```python
from build123d import *

# Parameters (mm, degrees)
EXTRUDE_1_DEPTH     = 2.121152063
SKETCH_2_W          = 18.284159781
SKETCH_2_H          = 2.121152063
EXTRUDE_2_DEPTH     = 1.283615947
SKETCH_3_W          = 7.715840219
SKETCH_3_H          = 2.121152063
EXTRUDE_3_DEPTH     = 1.283615947
EXTRUDE_4_DEPTH     = 4.2
SKETCH_5_W          = 31.999368794
SKETCH_5_H          = 4.790748137
EXTRUDE_5_DEPTH     = 2.1
SKETCH_6_W          = 12.000251863
SKETCH_6_H          = 4.2
CUT_EXTRUDE_1_DEPTH = 2.32
CUT_EXTRUDE_2_DEPTH = 23.550749058
EXTRUDE_6_DEPTH     = 3.1
EXTRUDE_7_DEPTH     = 3.1
CUT_EXTRUDE_3_DEPTH = 1
CUT_EXTRUDE_4_DEPTH = 2.6
CUT_EXTRUDE_5_DEPTH = 2.6
CUT_EXTRUDE_6_DEPTH = 0.7
CUT_EXTRUDE_7_DEPTH = 3.090748137
CUT_EXTRUDE_8_DEPTH = 3.090748137
HOLE_WIZARD_1_D     = 2.4
HOLE_WIZARD_1_DEPTH = 16.79105
HOLE_WIZARD_2_D     = 2.4
HOLE_WIZARD_2_DEPTH = 16.79105
HOLE_WIZARD_3_D     = 2.4
HOLE_WIZARD_3_DEPTH = 16.79105
HOLE_WIZARD_4_D     = 2.4
HOLE_WIZARD_4_DEPTH = 16.79105
FILLET_1_R          = 1
FILLET_2_R          = 1
FILLET_3_R          = 1
FILLET_4_R          = 1
FILLET_5_R          = 3
FILLET_6_R          = 3


with BuildPart() as part:
    # ｽｹｯﾁ1 → ﾎﾞｽ - 押し出し1 (new body)
    with BuildSketch(Plane.XZ.offset(24)):
        with BuildLine():
            Line((-17, 4.6), (-17, -10.907384053))
            Line((-17, -10.907384053), (1.284159781, -10.907384053))
            Line((1.284159781, -10.907384053), (1.284159781, -9.036499448))
            ThreePointArc((1.284159781, -9.036499448), (-3.636777298, -7.097679354), (-0.031629692, -3.227594621))
            ThreePointArc((-0.031629692, -3.227594621), (9.064370854, -1.683948584), (9.284159781, -10.907384053))
            Line((9.284159781, -10.907384053), (17, -10.907384053))
            Line((17, -10.907384053), (17, 4.6))
            Line((17, 4.6), (-17, 4.6))
        make_face()
    extrude(amount=-EXTRUDE_1_DEPTH)

    # ｽｹｯﾁ2 → ﾎﾞｽ - 押し出し2 (add)
    with BuildSketch(Plane(origin=(0, 0, -10.907384053), x_dir=(-1, 0, 0), z_dir=(0, 0, -1))):
        with Locations((7.85792011, -22.939423969)):
            Rectangle(SKETCH_2_W, SKETCH_2_H)
    extrude(amount=EXTRUDE_2_DEPTH)

    # ｽｹｯﾁ3 → ﾎﾞｽ - 押し出し3 (add)
    with BuildSketch(Plane(origin=(0, 0, -10.907384053), x_dir=(-1, 0, 0), z_dir=(0, 0, -1))):
        with Locations((-13.14207989, -22.939423969)):
            Rectangle(SKETCH_3_W, SKETCH_3_H)
    extrude(amount=EXTRUDE_3_DEPTH)

    # ｽｹｯﾁ4 → ﾎﾞｽ - 押し出し4 (add)
    with BuildSketch(Plane(origin=(0, -21.878847937, 0), x_dir=(-1, 0, 0), z_dir=(0, 1, 0))):
        with BuildLine():
            Line((17, 4.6), (17, -12.191))
            Line((17, -12.191), (11.515840219, -12.191))
            Line((11.515840219, -12.191), (11.515840219, -0.190748137))
            Line((11.515840219, -0.190748137), (-9.284159781, -0.190748137))
            Line((-9.284159781, -0.190748137), (-9.284159781, -12.191))
            add(Edge.make_bspline(
                [(-9.284159781, -12.191), (-10.057493115, -12.191), (-10.830826448, -12.191), (-11.604159781, -12.191)],
                knots=[0, 0, 0, 0, 1, 1, 1, 1], degree=3))
            Line((-11.604159781, -12.191), (-17, -12.191))
            Line((-17, -12.191), (-17, 4.6))
            Line((-17, 4.6), (17, 4.6))
        make_face()
    extrude(amount=EXTRUDE_4_DEPTH)

    # ｽｹｯﾁ5 → ﾎﾞｽ - 押し出し5 (add)
    with BuildSketch(Plane(origin=(0, -17.678847937, 0), x_dir=(-1, 0, 0), z_dir=(0, 1, 0))):
        with Locations((-0.000159781, 2.204625932)):
            Rectangle(SKETCH_5_W, SKETCH_5_H)
    extrude(amount=EXTRUDE_5_DEPTH)

    # ｽｹｯﾁ6 → ｶｯﾄ - 押し出し1 (cut)
    with BuildSketch(Plane.ZY.offset(-9.284159781)):
        with Locations((-6.190874069, -19.778847937)):
            Rectangle(SKETCH_6_W, SKETCH_6_H)
    extrude(amount=-CUT_EXTRUDE_1_DEPTH, mode=Mode.SUBTRACT)

    # ｽｹｯﾁ7 → ｶｯﾄ - 押し出し2 (cut, through all)
    with BuildSketch(Plane.XZ.offset(24)):
        with BuildLine():
            Line((1.284159781, -11.081163897), (1.284159781, -9.036499448))
            ThreePointArc((1.284159781, -9.036499448), (0.655198078, -9.368779249), (-0.031629692, -9.553901653))
            ThreePointArc((-0.031629692, -9.553901653), (0.562738255, -10.37226331), (1.284159781, -11.081163897))
        make_face()
    extrude(amount=-CUT_EXTRUDE_2_DEPTH, mode=Mode.SUBTRACT)

    # ｽｹｯﾁ8 → ﾎﾞｽ - 押し出し6 (add)
    with BuildSketch(Plane(origin=(0, -17.678847937, 0), x_dir=(-1, 0, 0), z_dir=(0, 1, 0))):
        with BuildLine():
            Line((15.999524616, -6.990748137), (14.777524616, -6.990748137))
            ThreePointArc((14.777524616, -6.990748137), (12.865840219, -6.390748137), (14.777524616, -5.790748137))
            Line((14.777524616, -5.790748137), (15.999524616, -5.790748137))
            Line((15.999524616, -5.790748137), (15.999524616, -6.990748137))
        make_face()
    extrude(amount=EXTRUDE_6_DEPTH)

    # ｽｹｯﾁ9 → ﾎﾞｽ - 押し出し7 (add)
    with BuildSketch(Plane(origin=(0, -17.678847937, 0), x_dir=(-1, 0, 0), z_dir=(0, 1, 0))):
        with BuildLine():
            Line((-15.999844178, -5.790748137), (-14.745844178, -5.790748137))
            ThreePointArc((-14.745844178, -5.790748137), (-12.834159781, -6.390748137), (-14.745844178, -6.990748137))
            Line((-14.745844178, -6.990748137), (-15.999844178, -6.990748137))
            Line((-15.999844178, -6.990748137), (-15.999844178, -5.790748137))
        make_face()
    extrude(amount=EXTRUDE_7_DEPTH)

    # ｽｹｯﾁ10 → ｶｯﾄ - 押し出し3 (cut)
    with BuildSketch(Plane.XY.offset(4.6)):
        Polygon((-0.599999987, -17.799999602), (-2.834665696, -19.9353347), (-0.599999987, -22.159852817), (-0.599999987, -20.818248187), (2.589334329, -20.818248187), (2.589334329, -18.999999575), (-0.599999987, -18.999999575), align=None)
    extrude(amount=-CUT_EXTRUDE_3_DEPTH, mode=Mode.SUBTRACT)

    # ｽｹｯﾁ11 → ｶｯﾄ - 押し出し4 (cut)
    with BuildSketch(Plane.XY.offset(4.6)):
        Polygon((-14.535820787, -22.230633649), (-12.22641971, -22.230633649), (-11.071719172, -20.230633649), (-12.22641971, -18.230633649), (-14.535820787, -18.230633649), (-15.690521325, -20.230633649), align=None)
    extrude(amount=-CUT_EXTRUDE_4_DEPTH, mode=Mode.SUBTRACT)

    # ｽｹｯﾁ12 → ｶｯﾄ - 押し出し5 (cut)
    with BuildSketch(Plane.XY.offset(4.6)):
        Polygon((12.255035689, -22.231967066), (14.564436765, -22.231967066), (15.719137304, -20.231967066), (14.564436765, -18.231967066), (12.255035689, -18.231967066), (11.10033515, -20.231967066), align=None)
    extrude(amount=-CUT_EXTRUDE_5_DEPTH, mode=Mode.SUBTRACT)

    # ｽｹｯﾁ13 → ｶｯﾄ - 押し出し6 (cut)
    with BuildSketch(Plane(origin=(0, -21.878847937, 0), x_dir=(-1, 0, 0), z_dir=(0, 1, 0))):
        Polygon((7.518980495, -7.752475082), (5.003355584, -7.752475082), (5.003355584, -8.596713483), (8.530699304, -8.596713483), (8.530699304, -3.62698698), (7.518980495, -3.62698698), align=None)
    extrude(amount=-CUT_EXTRUDE_6_DEPTH, mode=Mode.SUBTRACT)

    # ｽｹｯﾁ14 → ｶｯﾄ - 押し出し7 (cut)
    with BuildSketch(Plane(origin=(0, 0, -0.190748137), x_dir=(-1, 0, 0), z_dir=(0, 0, -1))):
        Polygon((-7.185754105, -20.683997984), (-4.876353029, -20.683997984), (-3.72165249, -18.683997984), (-4.876353029, -16.683997984), (-7.185754105, -16.683997984), (-8.340454644, -18.683997984), align=None)
    extrude(amount=-CUT_EXTRUDE_7_DEPTH, mode=Mode.SUBTRACT)

    # ｽｹｯﾁ15 → ｶｯﾄ - 押し出し8 (cut)
    with BuildSketch(Plane(origin=(0, 0, -0.190748137), x_dir=(-1, 0, 0), z_dir=(0, 0, -1))):
        Polygon((4.835886318, -20.763995351), (7.145287395, -20.763995351), (8.299987933, -18.763995351), (7.145287395, -16.763995351), (4.835886318, -16.763995351), (3.68118578, -18.763995351), align=None)
    extrude(amount=-CUT_EXTRUDE_8_DEPTH, mode=Mode.SUBTRACT)

    # 穴1
    with Locations(Plane.XY.offset(4.6)):
        with Locations((-5.97769389, -18.770751676)):
            Hole(HOLE_WIZARD_1_D / 2, depth=HOLE_WIZARD_1_DEPTH)

    # 穴2
    with Locations(Plane.XY.offset(4.6)):
        with Locations((6.022013453, -18.686944197)):
            Hole(HOLE_WIZARD_2_D / 2, depth=HOLE_WIZARD_2_DEPTH)

    # 穴3
    with Locations(Plane(origin=(0, 0, -12.191), x_dir=(-1, 0, 0), z_dir=(0, 0, -1))):
        with Locations((-13.4, -20.25)):
            Hole(HOLE_WIZARD_3_D / 2, depth=HOLE_WIZARD_3_DEPTH)

    # 穴4
    with Locations(Plane(origin=(0, 0, -12.191), x_dir=(-1, 0, 0), z_dir=(0, 0, -1))):
        with Locations((13.4, -20.25)):
            Hole(HOLE_WIZARD_4_D / 2, depth=HOLE_WIZARD_4_DEPTH)

    # ﾌｨﾚｯﾄ1
    fillet_1_edges = [part.edges().sort_by_distance(p)[0] for p in [
        (9.284159781, -22.939423968, -10.907384053),
    ]]
    fillet(fillet_1_edges, radius=FILLET_1_R)

    # ﾌｨﾚｯﾄ2
    fillet_2_edges = [part.edges().sort_by_distance(p)[0] for p in [
        (1.284159781, -22.939423968, -11.081163897),
    ]]
    fillet(fillet_2_edges, radius=FILLET_2_R)

    # ﾌｨﾚｯﾄ3
    fillet_3_edges = [part.edges().sort_by_distance(p)[0] for p in [
        (-17, -17.678847937, -3.7955),
    ]]
    fillet(fillet_3_edges, radius=FILLET_3_R)

    # ﾌｨﾚｯﾄ4
    fillet_4_edges = [part.edges().sort_by_distance(p)[0] for p in [
        (17, -17.678847937, -3.7955),
    ]]
    fillet(fillet_4_edges, radius=FILLET_4_R)

    # ﾌｨﾚｯﾄ5
    fillet_5_edges = [part.edges().sort_by_distance(p)[0] for p in [
        (-17, -24, -3.7955),
    ]]
    fillet(fillet_5_edges, radius=FILLET_5_R)

    # ﾌｨﾚｯﾄ6
    fillet_6_edges = [part.edges().sort_by_distance(p)[0] for p in [
        (17, -24, -3.7955),
    ]]
    fillet(fillet_6_edges, radius=FILLET_6_R)


solid = part.part
```
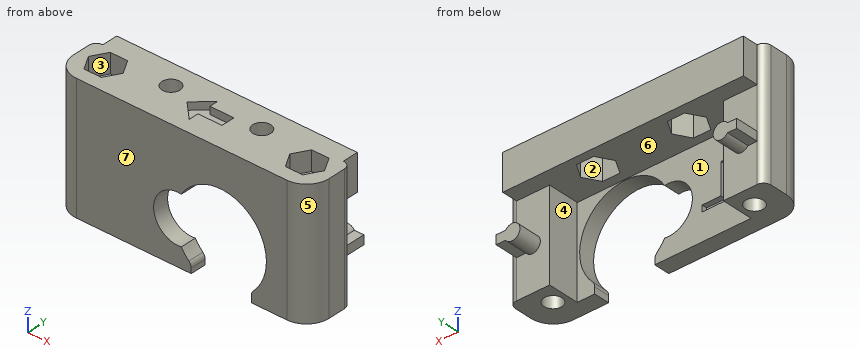
For this review, take the finished solid that the model builds, in its own axes (mm). Face numbers are marked on the shaded views. A direction names the side the tool comes from. Coordinates: 2 decimals unless noted, no trailing zeros. Write each loop counter-clockwise with the first axis right and the second up, starting at its lowest first coordinate (ties: lowest second). Pieces come first, ordered by that corner, then holes. Notation, with made-up numbers: (72.5, 42) -> (95.5, 42) arc R22 cw to (95.5, 78) -> close; hole circle Ø2 at (2, -35.75). An arc over 180 degrees is marked (long way). Put each result on its own line as item: value.
Q1. The part is to be moulded in two halves that separate along X. For the marked faces 4, 5, 6 and 7, say which applies: +X half, -X half, draft (parallel to the pull), parting line (faces both ways), or undercut.
From the geometry:
face 4: undercut
face 5: +X half
face 6: undercut
face 7: draft
Q2. Take a section at B-B, the plane x = -6. State the section outline as (y, z) points, then the cut area to 3 significant figures.
From the geometry:
outline: (-24, -12.19) -> (-21.88, -12.19) -> (-21.88, -8.6) -> (-22.58, -8.6) -> (-22.58, -7.75) -> (-21.88, -7.75) -> (-21.88, -0.19) -> (-20.76, -0.19) -> (-20.76, 2.9) -> (-19.97, 2.9) -> (-19.97, 4.6) -> (-24, 4.6) -> close; (-17.57, 2.9) -> (-16.76, 2.9) -> (-16.76, -0.19) -> (-15.58, -0.19) -> (-15.58, 4.6) -> (-17.57, 4.6) -> close
area: 48.8 mm2
Q3. Take a section at D-D, the plane x = 13.4. State the section outline as (y, z) points.
From the geometry:
outline: (-24, -12.19) -> (-21.45, -12.19) -> (-21.45, 2) -> (-22.23, 2) -> (-22.23, 4.6) -> (-24, 4.6) -> close; (-19.05, -12.19) -> (-17.68, -12.19) -> (-17.68, -7.32) -> (-14.58, -7.32) -> (-14.58, -5.46) -> (-17.68, -5.46) -> (-17.68, -0.19) -> (-15.58, -0.19) -> (-15.58, 4.6) -> (-18.23, 4.6) -> (-18.23, 2) -> (-19.05, 2) -> close
Q4. Take a section at C-C, the plane z = 0.75. Count the separate pieces of the cut face and the enclosed holes in it, then the cut area to 3 significant figures.
From the geometry:
separate pieces: 1
enclosed holes: 4
area: 241 mm2
Q5. Tool access review of the marked faces 1, 2 and 3: name each direction out of +Z, -Z, +X, -X, +Y, -Y from which nothing blocks a thin tool from reaching the whole face with its end or side.
From the geometry:
face 1: -Z, +Y
face 2: -Z
face 3: +Z
Q6. Take a section at A-A, the plane y = -16. State the section outline as (x, z) points, then the cut area to 3 significant figures.
From the geometry:
outline: (-16, -6.99) -> (-14.78, -6.99) arc R1.05 ccw (long way) to (-14.78, -5.79) -> (-16, -5.79) -> close; (-16, -0.19) -> (16, -0.19) -> (16, 4.6) -> (-16, 4.6) -> close; (14.75, -6.99) -> (16, -6.99) -> (16, -5.79) -> (14.75, -5.79) arc R1.05 ccw (long way) to start
area: 163 mm2
Q7. Wall thickness on L1, parallel to X at y = -20.25, z = 3; L2, parallel to Z at x = 15, y = -15.75; L3, parallel to X at y = -19.5, z = -11: over which ranges is each line inside the solid? List them lowest first.
From the geometry:
L1: x = -17 to -15.68, -11.08 to 11.11, 15.71 to 17
L2: z = -6.99 to -5.79, -0.19 to 4.6
L3: x = -17 to -14.34, -12.46 to -11.52, 11.6 to 12.46, 14.34 to 17
Q8. Clearance check with flat-ended pins moving along their axes: pin 1 Ø4.5 at (x, y) = (-5, -19) entering from -Z; pin 2 Ø8 at (x, z) = (1, -8.5) entering from +Y; pin 3 Ø4 at (x, y) = (1.5, -20) entering from -Z; pin 4 Ø2 at (x, z) = (-14.5, -2) entering from +Y. State where each tip first meets the part, or that it passes through.
From the geometry:
pin 1: stops at z = -0.19
pin 2: stops at y = -21.88
pin 3: stops at z = -12.19
pin 4: stops at y = -17.68
